```python
from build123d import *

# Parameters (mm, degrees)
SKETCH1_R           = 15
BOSS_EXTRUDE1_DEPTH = 30
SKETCH2_R           = 2.5
BOSS_EXTRUDE2_DEPTH = 20
CUT_EXTRUDE2_DEPTH  = 30
CIRPATTERN2_COUNT   = 6


with BuildPart() as part:
    # Sketch1 → Boss-Extrude1 (new, symmetric)
    with BuildSketch(Plane.XY):
        with Locations(Location((0, 0, 0), (0, 0, 180))):
            Circle(SKETCH1_R)
    extrude(amount=BOSS_EXTRUDE1_DEPTH, both=True)

    # Sketch2 → Boss-Extrude2 (add)
    with BuildSketch(Plane.XY.offset(30)):
        Circle(SKETCH2_R)
    extrude(amount=BOSS_EXTRUDE2_DEPTH)

    # Sketch4 → Cut-Extrude2 (cut)
    with BuildSketch(Plane.XY.offset(30)):
        with BuildLine():
            Line((-4.788282007, 13.155696691), (-5.13030215, 14.095389312))
            ThreePointArc((-5.13030215, 14.095389312), (0, 15), (5.13030215, 14.095389312))
            Line((5.13030215, 14.095389312), (4.788282007, 13.155696691))
            ThreePointArc((4.788282007, 13.155696691), (0, 14), (-4.788282007, 13.155696691))
        make_face()
    cut_extrude2 = extrude(amount=-CUT_EXTRUDE2_DEPTH, mode=Mode.SUBTRACT)

    # CirPattern2: Cut-Extrude2 ×6 about axis
    cirpattern2_axis = Axis((0, 0, 0), (0, 0, 1))
    for i in range(1, CIRPATTERN2_COUNT):
        add(cut_extrude2.rotate(cirpattern2_axis, i * 360 / CIRPATTERN2_COUNT), mode=Mode.SUBTRACT)


solid = part.part
```
Check sheet for the modelled part. Datum: model origin and axes. Units: mm. A direction names the side the tool comes from. Coordinates: 2 decimals unless noted, no trailing zeros. Write each loop counter-clockwise with the first axis right and the second up, starting at its lowest first coordinate (ties: lowest second). Pieces come first, ordered by that corner, then holes. Notation, with made-up numbers: (3.25, -29.5) - (32.25, -29.5) arc R32 ccw to (32.25, 9.5) - close; hole circle Ø7 at (-37, 49). An arc over 180 degrees is marked (long way). One line per question, with ' | ' between items.
Item 1: Sectioned sample at C-C on y = 7.5. Record the boundary of the cut face in (x, z), plus the area to 3 significant figures.
Determined:
outline: (-12.99, -30) - (12.99, -30) - (12.99, 0) - (11.82, 0) - (11.82, 30) - (-11.82, 30) - (-11.82, 0) - (-12.99, 0) - close | area: 1,490 mm2
Item 2: Gauge pin test, flat ends, axial feed: P1, Ø2, axis at y = -12, z = 28, coming from the -X side; P2, Ø0.6, axis at x = 2, y = -14.5, coming from the +Z side; P3, Ø1.7, axis at x = -11, y = -7, coming from the +Z side. Record the tip position at first contact, or that the pin passes through.
Determined:
P1: stops at x = -9.64 | P2: stops at z = 0 | P3: stops at z = 30
Item 3: Mould release check, pull along X, two halves, no side actions. Record for faces 5 (the face through (0, 0, -30)), 6 (the face through (0.1, 14.3, 0)), 7 (the face through (-6.92, 13.31, -6.25)): pulls with the +X half, pulls with the -X half, needs draft (parallel to the pull), parting line crosses it, or undercut.
Determined:
face 5: needs draft | face 6: undercut | face 7: parting line crosses it
Item 4: Access from +Z, -Z, +X, -X, +Y, -Y to the whole of each face (thin tool, end or side, straight path). Record for faces 1 (the face through (0, 0, 50)), 2 (the face through (-0.54, -2.44, 39.86)), 3 (the face through (0, 14, 15)), 4 (the face through (-0.1, -14.3, 0)).
Determined:
face 1: +Z, +X, -X, +Y, -Y | face 2: +Z | face 3: +Z, +Y | face 4: +Z, -Y
Item 5: Thickness scan on line 1 (Y direction, x = -10.5, z = -21.5); line 2 (Z direction, x = 2.75, y = 12.75); line 3 (Y direction, x = -0.5, z = 16). Record the ranges inside material, lowest first. Write a range as [from, to].
Determined:
line 1: y = [-10.71, 10.71] | line 2: z = [-30, 30] | line 3: y = [-13.99, 13.99]
Item 6: Sectioned sample at D-D on y = 0. Record the boundary of the cut face in (x, z).
Determined:
outline: (-15, -30) - (15, -30) - (15, 30) - (2.5, 30) - (2.5, 50) - (-2.5, 50) - (-2.5, 30) - (-15, 30) - close
Item 7: Sectioned sample at A-A on z = 2.5. Record the boundary of the cut face in (x, y), plus the area to 3 significant figures.
Determined:
outline: (-14.77, -2.6) - (-13.79, -2.43) arc R14 ccw to (-9, -10.72) - (-9.64, -11.49) arc R15 ccw to (-5.13, -14.1) - (-4.79, -13.16) arc R14 ccw to (4.79, -13.16) - (5.13, -14.1) arc R15 ccw to (9.64, -11.49) - (9, -10.72) arc R14 ccw to (13.79, -2.43) - (14.77, -2.6) arc R15 ccw to (14.77, 2.6) - (13.79, 2.43) arc R14 ccw to (9, 10.72) - (9.64, 11.49) arc R15 ccw to (5.13, 14.1) - (4.79, 13.16) arc R14 ccw to (-4.79, 13.16) - (-5.13, 14.1) arc R15 ccw to (-9.64, 11.49) - (-9, 10.72) arc R14 ccw to (-13.79, 2.43) - (-14.77, 2.6) arc R15 ccw to start | area: 646 mm2
Item 8: Sectioned sample at B-B on x = 0. Record the boundary of the cut face in (y, z).
Determined:
outline: (-15, -30) - (15, -30) - (15, 0) - (14, 0) - (14, 30) - (2.5, 30) - (2.5, 50) - (-2.5, 50) - (-2.5, 30) - (-14, 30) - (-14, 0) - (-15, 0) - close
